Could you check a few things on this model? Use its own coordinates, in mm. Face numbers are marked on the shaded views. Round coordinates to 2 decimals unless told otherwise and drop trailing zeros. Loops run counter-clockwise (first coordinate to the right, second up) from the corner with the lowest first, then second, coordinate; pieces in that order, holes last.
Autodesk Inventor part; units mm, degrees
ref_plane "YZ Plane" through (0, 0, 0) normal (1, 0, 0) x (0, 1, 0)
ref_plane "XZ Plane" through (0, 0, 0) normal (0, 1, 0) x (-1, 0, 0)
ref_plane "XY Plane" through (0, 0, 0) normal (0, 0, 1) x (1, 0, 0)
sketch "Sketch1" plane through (0, 0, 0) normal (0, 0, 1) x (1, 0, 0)
  line L0 (-20, -4) -> (20, -4)
  line L1 (20, -4) -> (20, 4)
  line L2 (20, 4) -> (-20, 4)
  line L3 (-20, 4) -> (-20, -4)
  line L4 (-20, -4) -> (20, 4) construction
  line L5 (20, -4) -> (-20, 4) construction
  point P0 (0, 0)
  dimension "d0" = 8
  dimension "d1" = 40
extrude "Extrusion1" add sketch "Sketch1" along normal blind 8
sketch "Sketch2" plane through (-20, -4, 0) normal (0, -1, 0) x (1, 0, 0)
  line L0 (0, 0) -> (40, 0)
  line L1 (40, 0) -> (40, 8)
  line L2 (0, 8) -> (40, 8)
  line L3 (0, 0) -> (0, 8)
  point P0 (20, 0)
extrude "Extrusion2" add sketch "Sketch2" along normal blind 5
sketch "Sketch3" plane through (0, 0, 8) normal (0, 0, 1) x (1, 0, 0)
  line L0 (-15, -3) -> (15, -3) construction
  line L1 (15, -3) -> (15, 3) construction
  line L2 (15, 3) -> (-15, 3) construction
  line L3 (-15, 3) -> (-15, -3) construction
  line L4 (-15, -3) -> (15, 3) construction
  line L5 (15, -3) -> (-15, 3) construction
  line L6 (-28, 0) -> (28, 0)
  circle A0 centre (-9, 0) radius 2.65
  point P0 (0, 0)
  dimension "d6" = 6
  dimension "d7" = 30
  dimension "d8" = 5.3
extrude "Extrusion3" cut sketch "Sketch3" against normal through all
sketch "Sketch4" plane through (0, 0, 8) normal (0, 0, 1) x (1, 0, 0)
  line L0 (-13, -2.5) -> (13, -2.5)
  line L1 (13, -2.5) -> (13, 2.5)
  line L2 (13, 2.5) -> (-13, 2.5)
  line L3 (-13, 2.5) -> (-13, -2.5)
  line L4 (-13, -2.5) -> (13, 2.5) construction
  line L5 (13, -2.5) -> (-13, 2.5) construction
  circle A0 centre (-9, 0) radius 2.65
  point P0 (0, 0)
  point P1 (-8.1211, 2.5)
  point P2 (-8.1211, -2.5)
  point P3 (-9.8789, -2.5)
  point P4 (-9.8789, 2.5)
  dimension "d11" = 26
  dimension "d12" = 5
extrude "Extrusion4" add sketch "Sketch4" along normal blind 1.5 contours L3 L2 A0 L0 | A0 L2 L1 L0
fillet "Fillet1" radius 1 4 edges at (-9.8789, -2.5, 8.75) (-9.8789, 2.5, 8.75) (-8.1211, -2.5, 8.75) (-8.1211, 2.5, 8.75)
fillet "Fillet2" radius 2 4 edges at (-20, -9, 4) (-20, 4, 4) (20, -9, 4) (20, 4, 4)
chamfer "Chamfer1" distance 0.5 angle 45 9 edges at (0, -9, 0) (19.4142, -8.4142, 0) (20, -2.5, 0) (19.4142, 3.4142, 0) (0, 4, 0) (-19.4142, 3.4142, 0) (-20, -2.5, 0) (-19.4142, -8.4142, 0) (-11.65, 0, 0)
properties part number "SideHolderFix1"
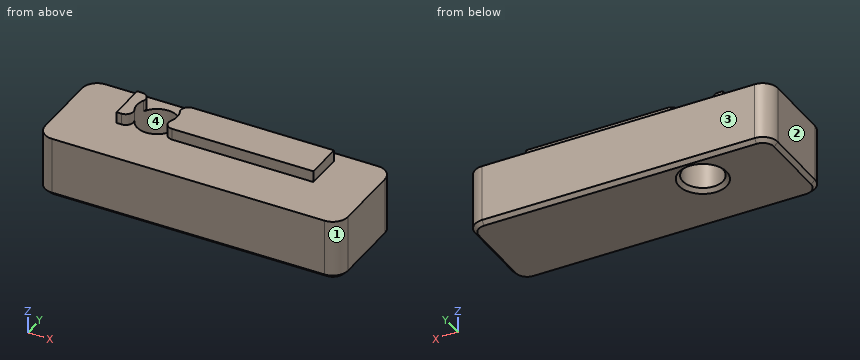
Item 1: If I drill on line 1 along X through (y, z) = (0, 4.75); line 2 along Y through (x, z) = (-9, 4.25); line 3 along Z through (x, y) = (7, -8), over which ranges is the centre line in solid material (lowest first)?
Results list:
line 1: x = -20 to -11.65, -6.35 to 20
line 2: y = -9 to -2.65, 2.65 to 4
line 3: z = 0 to 8
Item 2: If we section it at D-D, the plane x = 0: Please give me the cut outline in (y, z).
Results list:
outline: (-9, 0.5) - (-8.5, 0) - (3.5, 0) - (4, 0.5) - (4, 8) - (2.5, 8) - (2.5, 9.5) - (-2.5, 9.5) - (-2.5, 8) - (-9, 8) - close
Item 3: If we section it at A-A, the plane y = 0: Please give me the cut outline in (x, z).
Results list:
outline: (-20, 0.5) - (-19.5, 0) - (-12.15, 0) - (-11.65, 0.5) - (-11.65, 9.5) - (-13, 9.5) - (-13, 8) - (-20, 8) - close; (-6.35, 0.5) - (-5.85, 0) - (19.5, 0) - (20, 0.5) - (20, 8) - (13, 8) - (13, 9.5) - (-6.35, 9.5) - close
Item 4: We'd pull the mould along X, two halves only. Please class the marked faces 1, 2, 3 and 4: released by +X, released by -X, zero draft, split by the parting line, or undercut.
Results list:
face 1: released by +X
face 2: released by -X
face 3: zero draft
face 4: undercut
Item 5: If we section it at C-C, the plane z = 5.75: Please give me the cut outline in (x, y).
Results list:
outline: (-20, -7) arc R2 ccw to (-18, -9) - (18, -9) arc R2 ccw to (20, -7) - (20, 2) arc R2 ccw to (18, 4) - (-18, 4) arc R2 ccw to (-20, 2) - close; hole circle Ø5.3 at (-9, 0)
Item 6: If we section it at B-B, the plane x = -9: Please give me the cut outline in (y, z).
Results list:
outline: (-9, 0.5) - (-8.5, 0) - (-3.15, 0) - (-2.65, 0.5) - (-2.65, 8) - (-9, 8) - close; (2.65, 0.5) - (3.15, 0) - (3.5, 0) - (4, 0.5) - (4, 8) - (2.65, 8) - close
Item 7: Will these pins go through, and if not, where does the flat tip stop? pin 1 (0.8 mm diameter, centred on y = 0, z = 8.5, fed in from +X); pin 2 (1.6 mm diameter, centred on x = 7, z = 9, fed in from +Y); pin 3 (0.8 mm diameter, centred on y = 0.5, z = 8.5, fed in from -X).
Results list:
pin 1: stops at x = 13
pin 2: stops at y = 2.5
pin 3: stops at x = -13
